from build123d import *

# Parameters (mm, degrees)
SKETCH_1_W            = 115
SKETCH_1_H            = 119.4
EXTRUDE_1_DEPTH       = 5
SKETCH_2_W            = 20
SKETCH_2_H            = 4
SKETCH_2_W_2          = 34
EXTRUDE_2_DEPTH       = 20
F_3_0MM_1_D           = 3
F_3_0MM_1_CSINK_D     = 3.05
F_3_0MM_1_CSINK_ANGLE = 90
FILLET_1_R            = 10
FILLET_2_R            = 5
FILLET_3_R            = 5
SKETCH_5_R            = 1.5
SKETCH_5_R_2          = 1.499237998
SKETCH_5_R_3          = 1.65
CUT_EXTRUDE_1_DEPTH   = 106.373307238
CUT_EXTRUDE_2_DEPTH   = 106.373307262


with BuildPart() as part:
    # 草图1 → 凸台-拉伸1 (new body)
    with BuildSketch(Plane.XY):
        with Locations((25.302465961, 0.485426053)):
            Rectangle(SKETCH_1_W, SKETCH_1_H)
    extrude(amount=EXTRUDE_1_DEPTH)

    # 草图2 → 凸台-拉伸2 (add)
    with BuildSketch(Plane(origin=(0, 0, 0), x_dir=(-1, 0, 0), z_dir=(0, 0, -1))):
        with Locations((22.197534039, 52.385426053)):
            Rectangle(SKETCH_2_W, SKETCH_2_H)
        with Locations((-65.802465961, 52.385426053)):
            Rectangle(SKETCH_2_W_2, SKETCH_2_H)
        with Locations((-65.802465961, -51.414573947)):
            Rectangle(SKETCH_2_W_2, SKETCH_2_H)
        with Locations((22.197534039, -51.414573947)):
            Rectangle(SKETCH_2_W, SKETCH_2_H)
    extrude(amount=EXTRUDE_2_DEPTH)

    # Ø3.0mm 暗销孔1 (through all)
    with Locations(Plane(origin=(0, 54.385426053, 0), x_dir=(1, 0, 0), z_dir=(0, 1, 0))):
        with Locations((62, 15), (-16.57, 15), (-26.57, 15), (52, 15)):
            CounterSinkHole(F_3_0MM_1_D / 2, F_3_0MM_1_CSINK_D / 2, counter_sink_angle=F_3_0MM_1_CSINK_ANGLE)

    # 圆角1
    fillet_1_edges = [part.edges().sort_by_distance(p)[0] for p in [
        (82.802465961, 52.385426053, -20),
        (82.802465961, -51.414573947, -20),
    ]]
    fillet(fillet_1_edges, radius=FILLET_1_R)

    # 圆角2
    fillet_2_edges = [part.edges().sort_by_distance(p)[0] for p in [
        (-12.197534039, 52.385426053, -20),
        (-32.197534039, 52.385426053, -20),
        (48.802465961, 52.385426053, -20),
        (48.802465961, -51.414573947, -20),
        (-12.197534039, -51.414573947, -20),
        (-32.197534039, -51.414573947, -20),
    ]]
    fillet(fillet_2_edges, radius=FILLET_2_R)

    # 圆角3
    fillet_3_edges = [part.edges().sort_by_distance(p)[0] for p in [
        (-32.197534039, 60.185426053, 2.5),
        (82.802465961, 60.185426053, 2.5),
        (82.802465961, -59.214573947, 2.5),
        (-32.197534039, -59.214573947, 2.5),
    ]]
    fillet(fillet_3_edges, radius=FILLET_3_R)

    # 草图5 → 切除-拉伸1 (cut, through all)
    with BuildSketch(Plane.XY.offset(5)):
        with Locations((-33.10026153, 49.4399256)):
            Circle(SKETCH_5_R)
        with Locations((20.89973847, 49.439163598)):
            Circle(SKETCH_5_R_2)
        with Locations((20.89973847, 0.4399256)):
            Circle(SKETCH_5_R)
        with Locations((-33.10026153, 0.4399256)):
            Circle(SKETCH_5_R)
        with Locations((59.875063234, 42.198126078)):
            Circle(SKETCH_5_R)
        with Locations((75.875063234, 42.198126078)):
            Circle(SKETCH_5_R)
        with Locations((59.875063234, -41.801873922)):
            Circle(SKETCH_5_R)
        with Locations((75.875063234, -41.801873922)):
            Circle(SKETCH_5_R)
        with Locations((-33.346706732, -42.112908038)):
            Circle(SKETCH_5_R_3)
        with Locations((-33.346706732, -10.412908038)):
            Circle(SKETCH_5_R_3)
        with Locations((24.353293268, -10.412908038)):
            Circle(SKETCH_5_R_3)
        with Locations((24.353293268, -42.112908038)):
            Circle(SKETCH_5_R_3)
    extrude(amount=-CUT_EXTRUDE_1_DEPTH, mode=Mode.SUBTRACT)

    # 草图6 → 切除-拉伸2 (cut, through all)
    with BuildSketch(Plane.XY.offset(5)):
        with BuildLine():
            Line((-5.197534039, -8.214573947), (26.802465961, -8.214573947))
            ThreePointArc((26.802465961, -8.214573947), (27.802465961, -9.214573947), (26.802465961, -10.214573947))
            Line((26.802465961, -10.214573947), (-5.197534039, -10.214573947))
            ThreePointArc((-5.197534039, -10.214573947), (-6.197534039, -9.214573947), (-5.197534039, -8.214573947))
        make_face()
        with BuildLine():
            Line((-5.197534039, -45.214573947), (26.802465961, -45.214573947))
            ThreePointArc((26.802465961, -45.214573947), (27.802465961, -46.214573947), (26.802465961, -47.214573947))
            Line((26.802465961, -47.214573947), (-5.197534039, -47.214573947))
            ThreePointArc((-5.197534039, -47.214573947), (-6.197534039, -46.214573947), (-5.197534039, -45.214573947))
        make_face()
    extrude(amount=-CUT_EXTRUDE_2_DEPTH, mode=Mode.SUBTRACT)


solid = part.part
CAD build for the part. Positions are in the model's coordinates, mm. A direction names the side the tool comes from. Give positions to 0.01 mm unless a question says otherwise; leave off trailing zeros. Loops run counter-clockwise (first coordinate to the right, second up) from the corner with the lowest first, then second, coordinate; pieces in that order, holes last. Notation, with made-up numbers: M 33,-5.5 L 43,-5.5 A25 cw 43,11.5 Z; hole C 47.5,69.25 d6. An arc over 180 degrees is marked long. Answer in a Markdown table with one row per item. Add a question column.
Item 1: Probe probe 1 along Y at (x, z) = (76, 2); probe 2 along Y at (x, z) = (26.5, 2.5); probe 3 along Y at (x, z) = (68, -5). List the from-to ranges inside material, lowest first.
Item 2: Band-saw the part on C-C on y = -51. Give the cut face in (x, z), then the cut area to 3 significant figures.
Item 3: Band-saw the part on D-D on x = 52. Give the cut face in (y, z) (3 decimals).
Item 4: Mould opens along Z. For faces 1 (the face through (81.38, 58.68, 2.54)), 2 (the face through (79.795, 52.413, -17.148)), 3 (the face through (60.57, 52.35, -15.45)) say: +Z half, -Z half, draft (parallel to the pull), parting line (faces both ways), or undercut.
Item 5: Band-saw the part on A-A on z = -3. Give the cut face in (x, y).
Item 6: Tool access for faces 4 (the face through (48.802, -51, -7)), 5 (the face through (66, 50.385, -10)), 6 (the face through (24, 1, 5)), 7 (the face through (66, -53.415, -10)): list every direction of +Z, -Z, +X, -X, +Y, -Y with a clear straight run to the whole face (end or side of a thin tool).
Item 7: Band-saw the part on B-B on x = 17. Give the cut face in (y, z).
Item 8: Drop flat-ended pins along their axis: P1, Ø5.5, axis at x = 24.35, y = -42.11, coming from the -Z side; P2, Ø2.5, axis at x = -16.57, z = -15, coming from the -Y side; P3, Ø4.5, axis at x = 24.35, y = -10.41, coming from the +Z side; P4, Ø6, axis at x = 68.5, z = -13.5, coming from the -Y side. Give the stop position or say it passes through.
Reply:
| question | item | result |
|---|---|---|
| 1 | probe 1 | y = -59.21 to -43.3, -40.31 to 40.7, 43.69 to 60.19 |
| 1 | probe 2 | y = -59.21 to -47.21, -45.21 to -10.21, -8.21 to 60.19 |
| 1 | probe 3 | y = -53.41 to -49.41, 50.39 to 54.39 |
| 2 | outline | M -32.2,-15 A5 ccw -27.2,-20 L -17.2,-20 A5 ccw -12.2,-15 L -12.2,0 L 48.8,0 L 48.8,-15 A5 ccw 53.8,-20 L 72.8,-20 A10 ccw 82.8,-10 L 82.8,5 L -32.2,5 Z; hole C -26.57,-15 d3; hole C -16.57,-15 d3; hole C 52,-15 d3; hole C 62,-15 d3 |
| 2 | area | 1,590 mm^2 |
| 3 | outline | M -59.215,0 L -53.415,0 L -53.415,-13.5 L -49.415,-13.5 L -49.415,0 L 50.385,0 L 50.385,-13.5 L 54.36,-13.5 L 54.385,-13.475 L 54.385,0 L 60.185,0 L 60.185,5 L -59.215,5 Z; M -53.415,-19.664 L -49.415,-19.664 L -49.415,-16.5 L -53.415,-16.5 Z; M 50.385,-19.664 L 54.385,-19.664 L 54.385,-16.525 L 54.36,-16.5 L 50.385,-16.5 Z |
| 4 | face 1 | draft |
| 4 | face 2 | -Z half |
| 4 | face 3 | undercut |
| 5 | outline | M -32.2,-53.41 L -12.2,-53.41 L -12.2,-49.41 L -32.2,-49.41 Z; M -32.2,50.64 A1.5 cw -31.94,50.39 L -12.2,50.39 L -12.2,54.39 L -32.2,54.39 Z; M 48.8,-53.41 L 82.8,-53.41 L 82.8,-49.41 L 48.8,-49.41 Z; M 48.8,50.39 L 82.8,50.39 L 82.8,54.39 L 48.8,54.39 Z |
| 6 | face 4 | -Z, +Y, -Y |
| 6 | face 5 | -Z, +X, -X |
| 6 | face 6 | +Z, +X, -X, +Y, -Y |
| 6 | face 7 | -Z, +X, -X, -Y |
| 7 | outline | M -59.21,0 L -47.21,0 L -47.21,5 L -59.21,5 Z; M -45.21,0 L -10.21,0 L -10.21,5 L -45.21,5 Z; M -8.21,0 L 60.19,0 L 60.19,5 L -8.21,5 Z |
| 8 | P1 | stops at z = 0 |
| 8 | P2 | passes through |
| 8 | P3 | stops at z = 5 |
| 8 | P4 | stops at y = -53.41 |
